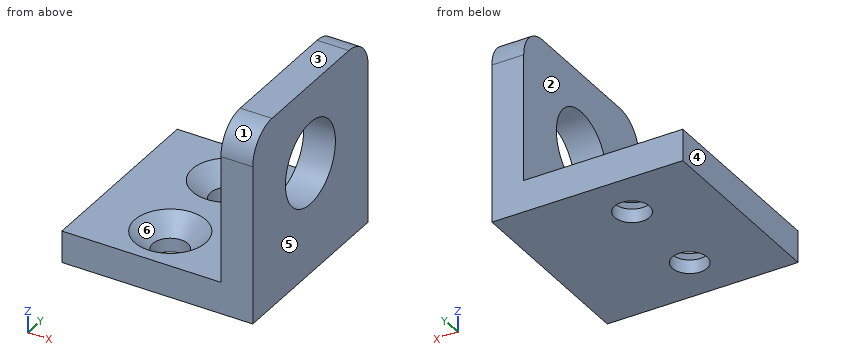
```python
from build123d import *

# Parameters (mm, degrees)
F1_DEPTH       = 30
F2_R           = 5
F3_R           = 6.5
F4_DEPTH       = 5.001
F6_D           = 5.5
F6_DEPTH       = 18
F6_CSINK_D     = 11.2
F6_CSINK_ANGLE = 90
F6_TIP         = 1.6523667023


with BuildPart() as f1:
    # F0 (on Front) → F1 (new body)
    with BuildSketch(Plane.XZ):
        Polygon((-15, -2.5), (15, -2.5), (15, 2.5), (15, 27.5), (10, 27.5), (10, 2.5), (-15, 2.5), align=None)
    extrude(amount=F1_DEPTH)

    # F2
    f2_edges = [f1.edges().sort_by_distance(p)[0] for p in [
        (12.5, 0, 27.5),
        (12.5, -30, 27.5),
    ]]
    fillet(f2_edges, radius=F2_R)

    # F3 (on face) → F4 (cut, through all)
    with BuildSketch(Plane(origin=(10, 0, 0), x_dir=(0, -1, 0), z_dir=(-1, 0, 0))):
        with Locations((15, 15)):
            Circle(F3_R)
    extrude(amount=-F4_DEPTH, mode=Mode.SUBTRACT)

    # F6
    with Locations(Plane.XY.offset(2.5)):
        with Locations((-2.5, -22.5), (-2.5, -7.5)):
            CounterSinkHole(F6_D / 2, F6_CSINK_D / 2, depth=F6_DEPTH, counter_sink_angle=F6_CSINK_ANGLE)
            with Locations((0, 0, -(F6_DEPTH + F6_TIP / 2))):  # 118° drill point
                Cone(0, F6_D / 2, F6_TIP, mode=Mode.SUBTRACT)


solid = f1.part
```
Source: CAD feature listing. Evaluate the final solid. Frame: model axes, mm. Face numbers are marked on the shaded views. A direction names the side the tool comes from. Coordinates: 2 decimals unless noted, no trailing zeros. Write each loop counter-clockwise with the first axis right and the second up, starting at its lowest first coordinate (ties: lowest second). Pieces come first, ordered by that corner, then holes. Notation, with made-up numbers: (54.5, 76.25) -> (107.5, 76.25) arc R18 ccw to (107.5, 100.25) -> close; hole circle Ø5 at (30, -26). An arc over 180 degrees is marked (long way). Return JSON: item names as keys, results as strings. Group by question number.
1) Section query A-A, the plane y = -15. Return loops of the section in (x, z), plus the area to 3 significant figures.
2) Set-up query: the marked faces 1 and 2. Return all of +Z, -Z, +X, -X, +Y, -Y with unobstructed straight access to the full face (end or side cutting, diameter ignored); none if empty.
3) Contact query for flat-ended pins moving along their axis: P1, Ø6, axis at x = 1, y = -14, coming from the +Z side; P2, Ø5, axis at x = -2.5, y = -22.5, coming from the -Z side; P3, Ø12.5, axis at y = -16.5, z = 9.5, coming from the -X side. Output: stop coordinate, or through.
4) Ray query, line 1 along X through (y, z) = (-7.5, -1.9); line 2 along Z through (x, y) = (12.35, -15); line 3 along X through (y, z) = (-10.5, 23.25). Return the intervals inside material, ascending.
5) Section query B-B, the plane z = 14.25. Return loops of the section in (x, y).
6) Mould query, pull axis X, two halves, no side actions, for the marked faces 3, 4, 5 and 6. Classes: +X half, -X half, draft (parallel to the pull), parting line (faces both ways), or undercut.
7) Section query D-D, the plane z = 1.75. Return loops of the section in (x, y), plus the area to 3 significant figures.
8) Section query C-C, the plane x = -2.5. Return loops of the section in (y, z), plus the area to 3 significant figures.
From the geometry:
{
 "1": {"outline": "(-15, -2.5) -> (15, -2.5) -> (15, 8.5) -> (10, 8.5) -> (10, 2.5) -> (-15, 2.5) -> close; (10, 21.5) -> (15, 21.5) -> (15, 27.5) -> (10, 27.5) -> close", "area": "210 mm²"},
 "2": {"face 1": "+Z, +X, -X, -Y", "face 2": "+Z, -X, +Y, -Y"},
 "3": {"P1": "z = 2.5", "P2": "through", "P3": "x = 10"},
 "4": {"line 1": "-15 to -5.25, 0.25 to 15", "line 2": "-2.5 to 8.5, 21.5 to 27.5", "line 3": "10 to 15"},
 "5": {"outline": "(10, -30) -> (15, -30) -> (15, -21.46) -> (10, -21.46) -> close; (10, -8.54) -> (15, -8.54) -> (15, 0) -> (10, 0) -> close"},
 "6": {"face 3": "draft", "face 4": "-X half", "face 5": "+X half", "face 6": "undercut"},
 "7": {"outline": "(-15, -30) -> (15, -30) -> (15, 0) -> (-15, 0) -> close; hole circle Ø9.7 at (-2.5, -22.5); hole circle Ø9.7 at (-2.5, -7.5)", "area": "752 mm²"},
 "8": {"outline": "(-30, -2.5) -> (-25.25, -2.5) -> (-25.25, -0.35) -> (-28.1, 2.5) -> (-30, 2.5) -> close; (-19.75, -2.5) -> (-10.25, -2.5) -> (-10.25, -0.35) -> (-13.1, 2.5) -> (-16.9, 2.5) -> (-19.75, -0.35) -> close; (-4.75, -2.5) -> (0, -2.5) -> (0, 2.5) -> (-1.9, 2.5) -> (-4.75, -0.35) -> close", "area": "78.8 mm²"}
}
